from build123d import *

# Parameters (mm, degrees)
ESBO_O1_W                = 43.18
ESBO_O1_H                = 17.78
RESSALTO_EXTRUS_O1_DEPTH = 1
ESBO_O5_R                = 0.75
RESSALTO_EXTRUS_O5_DEPTH = 1
RESSALTO_EXTRUS_O5_TAPER = 28
RESSALTO_EXTRUS_O4_DEPTH = 1
ESBO_O6_W                = 9
ESBO_O6_H                = 7.5
RESSALTO_EXTRUS_O6_DEPTH = 3.5
ESBO_O7_R                = 1
CORTE_EXTRUS_O1_DEPTH    = 2
ESBO_O8_W                = 6.5
ESBO_O8_H                = 2.5
ESBO_O8_W_2              = 5
ESBO_O8_H_2              = 1
CORTE_EXTRUS_O2_DEPTH    = 7
FILETE1_R                = 0.5


with BuildPart() as part:
    # Esbo_o1 → Ressalto-extrus_o1 (new body)
    with BuildSketch(Plane(origin=(0, 0, 0), x_dir=(1, 0, 0), z_dir=(0, 1, 0))):
        Rectangle(ESBO_O1_W, ESBO_O1_H)
    extrude(amount=RESSALTO_EXTRUS_O1_DEPTH)

    # Esbo_o5 → Ressalto-extrus_o5 (add)
    with BuildSketch(Plane(origin=(0, 1, 0), x_dir=(1, 0, 0), z_dir=(0, 1, 0))):
        with Locations((-17.89, 7.75)):
            Circle(ESBO_O5_R)
        with Locations((-17.89, -7.75)):
            Circle(ESBO_O5_R)
    extrude(amount=RESSALTO_EXTRUS_O5_DEPTH, taper=RESSALTO_EXTRUS_O5_TAPER)

    # Esbo_o4 → Ressalto-extrus_o4 (add)
    with BuildSketch(Plane(origin=(0, 1, 0), x_dir=(1, 0, 0), z_dir=(0, 1, 0))):
        Polygon((-10.839747468, 0), (-5.89, 4.949747468), (-0.940252532, 0), (-5.89, -4.949747468), align=None)
    extrude(amount=RESSALTO_EXTRUS_O4_DEPTH)

    # Esbo_o6 → Ressalto-extrus_o6 (add)
    with BuildSketch(Plane(origin=(0, 1, 0), x_dir=(1, 0, 0), z_dir=(0, 1, 0))):
        with Locations((-19.09, 0)):
            Rectangle(ESBO_O6_W, ESBO_O6_H)
    extrude(amount=RESSALTO_EXTRUS_O6_DEPTH)

    # Esbo_o7 → Corte-extrus_o1 (cut, through all)
    with BuildSketch(Plane(origin=(0, 1, 0), x_dir=(1, 0, 0), z_dir=(0, 1, 0))):
        with Locations((-20.29, 7.59)):
            Circle(ESBO_O7_R)
        with Locations((-20.29, -7.59)):
            Circle(ESBO_O7_R)
        with Locations((20.29, -7.59)):
            Circle(ESBO_O7_R)
        with Locations((20.29, 7.59)):
            Circle(ESBO_O7_R)
    extrude(amount=-CORTE_EXTRUS_O1_DEPTH, mode=Mode.SUBTRACT)

    # Esbo_o8 → Corte-extrus_o2 (cut)
    with BuildSketch(Plane.ZY.offset(23.59)):
        with Locations((0, 2.75)):
            Rectangle(ESBO_O8_W, ESBO_O8_H)
        with Locations((0, 2.75)):
            Rectangle(ESBO_O8_W_2, ESBO_O8_H_2, mode=Mode.SUBTRACT)
    extrude(amount=-CORTE_EXTRUS_O2_DEPTH, mode=Mode.SUBTRACT)

    # Filete1
    filete1_edges = [part.edges().sort_by_distance(p)[0] for p in [
        (-19.09, 4.5, -3.75),
        (-19.09, 4.5, 3.75),
    ]]
    fillet(filete1_edges, radius=FILETE1_R)


solid = part.part
Read the model definition and answer for the solid it produces. Units are mm, in the model's axes. A direction names the side the tool comes from. Round coordinates to 2 decimals unless told otherwise and drop trailing zeros. Loops run counter-clockwise (first coordinate to the right, second up) from the corner with the lowest first, then second, coordinate; pieces in that order, holes last.
Q1. Section B-B on z = 2 is taken. Write down the section's boundary in (x, y).
Q2. Section C-C on x = -7.5 is taken. Write down the section's boundary in (y, z).
Q3. Each of these flat-tipped pins is pushed along its axis until it touches: pin 1 (1.5 mm diameter, centred on y = 3, z = 2.5, fed in from +X); pin 2 (2.5 mm diameter, centred on x = -19.5, y = 2.5, fed in from +Z); pin 3 (0.8 mm diameter, centred on x = -20.5, y = 3, fed in from -Z). Where does it stop, or does it pass through?
Q4. Consider probe 1 along X at (y, z) = (0.2, 7.59); probe 2 along Z at (x, y) = (20.29, 0.25); probe 3 along X at (y, z) = (3.7, 0). Determine where each line is inside the solid, lowest interval first.
Q5. Section A-A on x = -20.29 is taken. Write down the section's boundary in (y, z), and give its area (3 significant figures).
Q6. Determine the mould class of faces 1 (the face through (-23.59, 3, 0)), 2 (the face through (-8.4, 1.49, -2.44)), 3 (the face through (-3.38, 1.49, 2.44)), 4 (the face through (-0.3, 0.5, 8.89)) for opening direction X: released by +X, released by -X, zero draft, split by the parting line, or undercut.
Q7. Which of the six approach directions +Z, -Z, +X, -X, +Y, -Y give full straight-line access (tool end or side, diameter ignored) to faces 5 (the face through (-14.59, 3, 0)), 6 (the face through (-3.45, 1.49, -2.51)), 7 (the face through (-6, 2, 0)), 8 (the face through (-21.027, 0.507, -8.266)), 9 (the face through (-20, 3, 2.5))?
Q8. Section D-D on z = -1.75 is taken. Write down the section's boundary in (x, y), and give its area (3 significant figures).
Output:
1. outline: (-23.59, 1) - (-21.59, 1) - (-21.59, 0) - (21.59, 0) - (21.59, 1) - (-2.94, 1) - (-2.94, 2) - (-8.84, 2) - (-8.84, 1) - (-14.59, 1) - (-14.59, 4.5) - (-23.59, 4.5) - (-23.59, 4) - (-16.59, 4) - (-16.59, 3.25) - (-23.59, 3.25) - (-23.59, 2.25) - (-16.59, 2.25) - (-16.59, 1.5) - (-23.59, 1.5) - close
2. outline: (0, -8.89) - (1, -8.89) - (1, -3.34) - (2, -3.34) - (2, 3.34) - (1, 3.34) - (1, 8.89) - (0, 8.89) - close
3. pin 1: stops at x = -14.59
3. pin 2: stops at z = 3.75
3. pin 3: stops at z = -3.75
4. probe 1: x = -21.59 to -21.29, -19.29 to 19.29, 21.29 to 21.59
4. probe 2: z = -8.89 to -8.59, -6.59 to 6.59, 8.59 to 8.89
4. probe 3: x = -16.59 to -14.59
5. outline: (0, -8.89) - (1, -8.89) - (1, -8.59) - (0, -8.59) - close; (0, -6.59) - (1, -6.59) - (1, -3.75) - (4, -3.75) arc R0.5 ccw to (4.5, -3.25) - (4.5, 3.25) arc R0.5 ccw to (4, 3.75) - (1, 3.75) - (1, 6.59) - (0, 6.59) - close; (0, 8.59) - (1, 8.59) - (1, 8.89) - (0, 8.89) - close; (2.25, -2.5) - (3.25, -2.5) - (3.25, 2.5) - (2.25, 2.5) - close; hole (1.5, -3.25) - (4, -3.25) - (4, 3.25) - (1.5, 3.25) - close
5. area: 28.7 mm2
6. face 1: released by -X
6. face 2: undercut
6. face 3: released by +X
6. face 4: zero draft
7. face 5: +Z, -Z, +Y
7. face 6: -Z, +X, +Y
7. face 7: +Z, -Z, +X, +Y
7. face 8: +Y, -Y
7. face 9: -X
8. outline: (-23.59, 1) - (-21.59, 1) - (-21.59, 0) - (21.59, 0) - (21.59, 1) - (-2.69, 1) - (-2.69, 2) - (-9.09, 2) - (-9.09, 1) - (-14.59, 1) - (-14.59, 4.5) - (-23.59, 4.5) - (-23.59, 4) - (-16.59, 4) - (-16.59, 3.25) - (-23.59, 3.25) - (-23.59, 2.25) - (-16.59, 2.25) - (-16.59, 1.5) - (-23.59, 1.5) - close
8. area: 70.6 mm2
